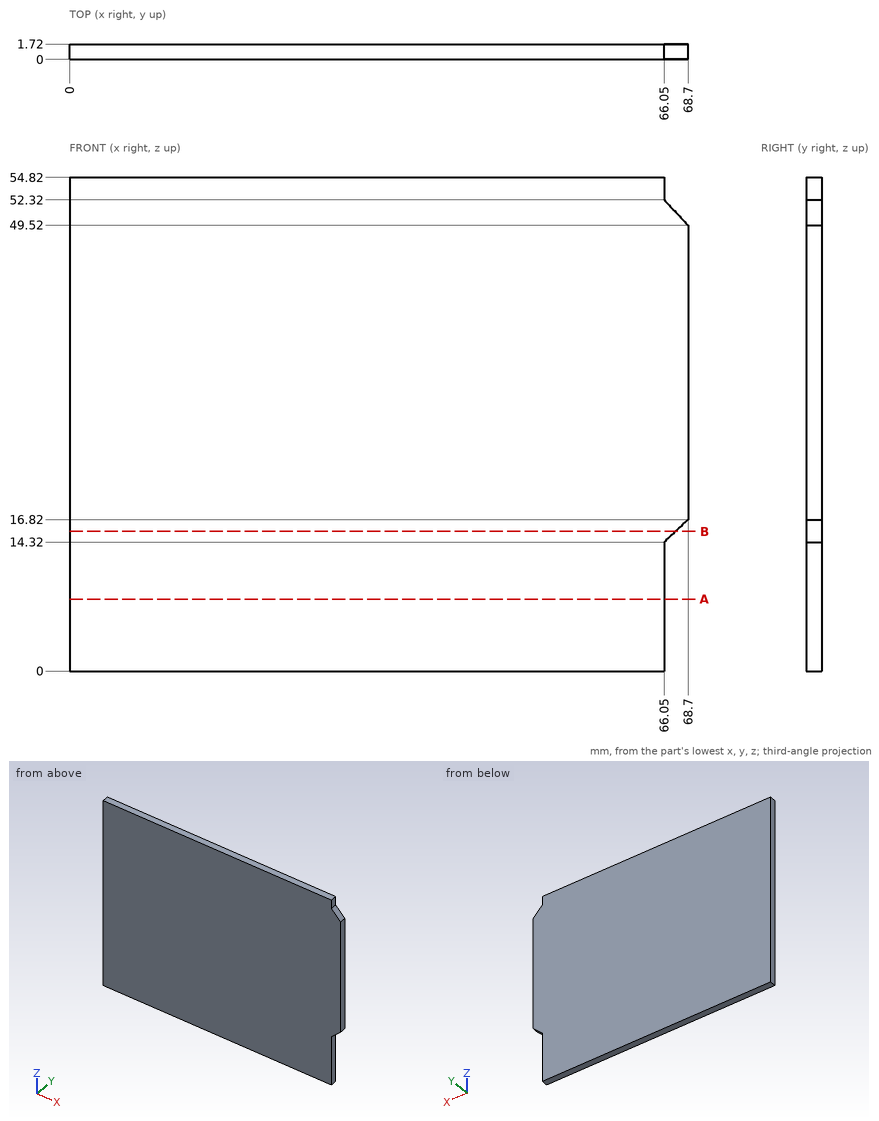
Part print with two shaded views. Sizes in mm from the minimum x, y, z corner. Coordinates: 2 decimals unless noted, no trailing zeros. Write each loop counter-clockwise with the first axis right and the second up, starting at its lowest first coordinate (ties: lowest second). Pieces come first, ordered by that corner, then holes.
1. Band-saw the part on A-A, the plane z = 8. Give the cut face in (x, y), and give its area (3 significant figures).
Answer block:
outline: (0, 0) - (66.05, 0) - (66.05, 1.72) - (0, 1.72) - close
area: 114 mm2
2. Drop a flat-ended pin along its axis: pin 1 (0.9 mm diameter, centred on y = 1, z = 54, fed in from +X). Give the stop position or say it passes through.
Answer block:
pin 1: stops at x = 66.05
3. Band-saw the part on B-B, the plane z = 15.5. Give the cut face in (x, y), and give its area (3 significant figures).
Answer block:
outline: (0, 0) - (67.3, 0) - (67.3, 1.72) - (0, 1.72) - close
area: 116 mm2
4. Drill centre lines: probe 1 along X at (y, z) = (0.1, 6.5); probe 2 along X at (y, z) = (1.45, 15). Where is each one in solid material? Low to high.
Answer block:
probe 1: x = 0 to 66.05
probe 2: x = 0 to 66.77
